Source: three-view drawing plus pictorial views. Frame: mm from the lowest corner of the part. Round coordinates to 2 decimals unless told otherwise and drop trailing zeros. Order: outer loops, then holes, each group sorted by start corner. A loop starts at its lowest first (then second) coordinate and runs counter-clockwise, first axis right, second up. Notation, with made-up numbers: (20.5, 77.5) -> (52.5, 77.5) arc R16 cw to (52.5, 102.5) -> close; hole circle Ø2 at (64, -14). An arc over 180 degrees is marked (long way). Answer as CSV lines item,"result". Start each with the question number.
1) Section query C-C, the plane z = 8. State how many separate pieces and enclosed holes the cut face has.
2) Mould query, pull axis X, two halves, no side actions, for the marked faces 1 and 2. Classes: +X half, -X half, draft (parallel to the pull), parting line (faces both ways), or undercut.
3) Line query: L1, parallel to X at y = 4.5, z = 9.25 (1 decimal); L2, parallel to X at y = 3, z = 6.75 (1 decimal); L3, parallel to Z at x = 10, y = 5.5 (1 decimal). Output: solid intervals per line, ascending.
4) Section query A-A, the plane z = 14.5. Output: boundary loops of the cut face in (x, y).
5) Section query B-B, the plane x = 62. Output: boundary loops of the cut face in (y, z).
6) First-contact query: P1, Ø8.5, axis at x = 9.525, z = 9.525, coming from the -Y side. Flat tip, straight axial feed; report the tip coordinate or a pass-through.
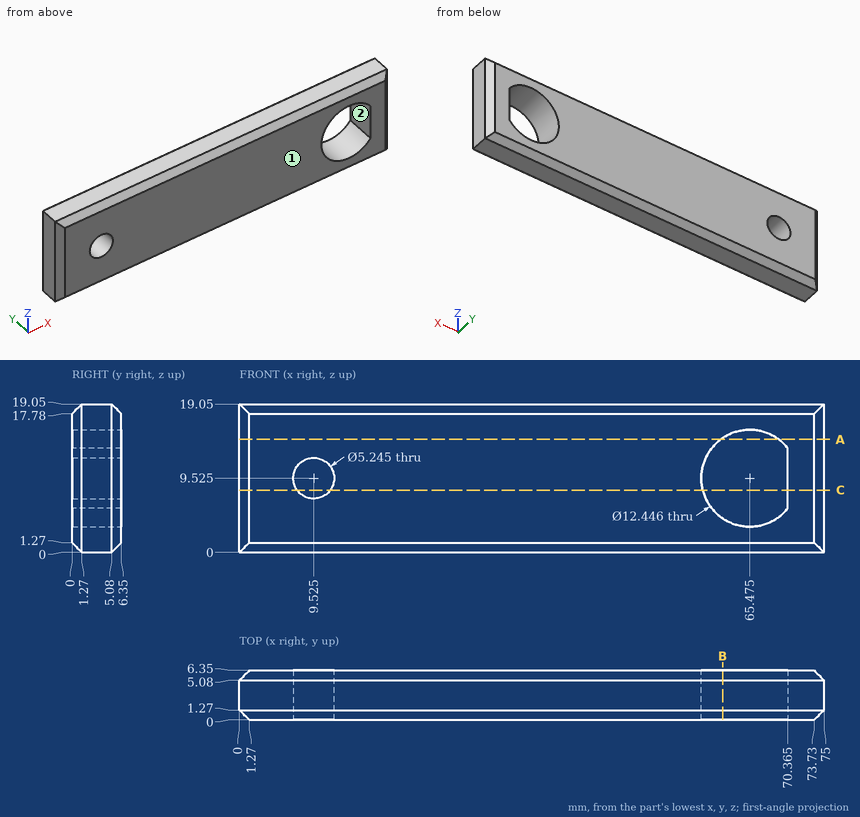
Findings:
1,separate pieces,"3"
1,enclosed holes,"0"
2,face 1,"draft"
2,face 2,"undercut"
3,L1,"x = 0 to 6.9, 12.1 to 59.3, 70.4 to 75"
3,L2,"x = 0 to 59.9, 70.4 to 75"
3,L3,"z = 0.4 to 6.9, 12.1 to 18.6"
4,outline,"(0, 1.27) -> (1.27, 0) -> (61.74, 0) -> (61.74, 6.35) -> (1.27, 6.35) -> (0, 5.08) -> close; (69.21, 0) -> (73.73, 0) -> (75, 1.27) -> (75, 5.08) -> (73.73, 6.35) -> (69.21, 6.35) -> close"
5,outline,"(0, 1.27) -> (1.27, 0) -> (5.08, 0) -> (6.35, 1.27) -> (6.35, 4.36) -> (0, 4.36) -> close; (0, 14.69) -> (6.35, 14.69) -> (6.35, 17.78) -> (5.08, 19.05) -> (1.27, 19.05) -> (0, 17.78) -> close"
6,P1,"stops at y = 0"
